For this review, take the finished solid that the model builds, in its own axes (mm). A direction names the side the tool comes from. Coordinates: 2 decimals unless noted, no trailing zeros. Loops run counter-clockwise (first coordinate to the right, second up) from the corner with the lowest first, then second, coordinate; pieces in that order, holes last. Notation, with made-up numbers: M 88,-7.75 L 123,-7.75 A20 cw 123,-1.75 Z; hole C 69,25 d3. An arc over 180 degrees is marked long. Write item = value, one per line.
from build123d import *

# Parameters (mm, degrees)
F0_R     = 2
F1_DEPTH = 32.8
F2_R     = 3
F3_DEPTH = 13.6
F4_DEPTH = 4


with BuildPart() as f1:
    # F0 (on Top) → F1 (new body)
    with BuildSketch(Plane.XY):
        with BuildLine():
            Line((77.5, 33.1), (-77.5, 33.1))
            ThreePointArc((-77.5, 33.1), (-84.571068, 30.171068), (-87.5, 23.1))
            Line((-87.5, 23.1), (-87.5, -23.1))
            ThreePointArc((-87.5, -23.1), (-84.571068, -30.171068), (-77.5, -33.1))
            Line((-77.5, -33.1), (77.5, -33.1))
            ThreePointArc((77.5, -33.1), (84.571068, -30.171068), (87.5, -23.1))
            Line((87.5, -23.1), (87.5, 23.1))
            ThreePointArc((87.5, 23.1), (84.571068, 30.171068), (77.5, 33.1))
        make_face()
        with Locations((-28.1, -20)):
            Circle(F0_R, mode=Mode.SUBTRACT)
        with Locations((71.9, -20)):
            Circle(F0_R, mode=Mode.SUBTRACT)
        with Locations((-28.1, 20)):
            Circle(F0_R, mode=Mode.SUBTRACT)
        with Locations((71.9, 20)):
            Circle(F0_R, mode=Mode.SUBTRACT)
        with Locations((-28.1, 20)):
            Circle(F0_R)
        with Locations((-28.1, -20)):
            Circle(F0_R)
        with Locations((71.9, 20)):
            Circle(F0_R)
        with Locations((71.9, -20)):
            Circle(F0_R)
    extrude(amount=F1_DEPTH)

    # F2 (on face) → F3 (join)
    with BuildSketch(Plane(origin=(-87.5, 0, 0), x_dir=(0, -1, 0), z_dir=(-1, 0, 0))):
        with Locations((0, 12)):
            Circle(F2_R)
    extrude(amount=F3_DEPTH)

    # F0 (on Top) → F4 (cut)
    with BuildSketch(Plane.XY):
        with Locations((-28.1, -20)):
            Circle(F0_R)
        with Locations((-28.1, 20)):
            Circle(F0_R)
        with Locations((71.9, 20)):
            Circle(F0_R)
        with Locations((71.9, -20)):
            Circle(F0_R)
    extrude(amount=F4_DEPTH, mode=Mode.SUBTRACT)


solid = f1.part
Q1. For pin 1 Ø1.2 at (x, y) = (-27, -20) entering from -Z; pin 2 Ø3 at (y, z) = (1.5, 25) entering from -X, all flat-tipped, find the tip position at first contact; note any pin that passes through.
Solved:
pin_1 = 4
pin_2 = -87.5
Q2. Add section B-B (y = -20). Write out the cut boundary in (x, z), and give its area (3 significant figures).
Solved:
outline = M -87.5,0 L -30.1,0 L -30.1,4 L -26.1,4 L -26.1,0 L 69.9,0 L 69.9,4 L 73.9,4 L 73.9,0 L 87.5,0 L 87.5,32.8 L -87.5,32.8 Z
area = 5,710 mm²
Q3. For line 1 along Y through (x, z) = (-28.1, 1.45); line 2 along X through (y, z) = (11, 27.5); line 3 along Y through (x, z) = (71, 1), list the stretches that pass through material, from the lowest coordinate up.
Solved:
line_1 = -33.1 to -22, -18 to 18, 22 to 33.1
line_2 = -87.5 to 87.5
line_3 = -33.1 to -21.79, -18.21 to 18.21, 21.79 to 33.1
Q4. Machinability: for faces 1 (the face through (-84.65, -30.09, 16.17)), 2 (the face through (-28, -20, 4)), 3 (the face through (-94.2, 0.65, 9.07)), which of the approach directions +Z, -Z, +X, -X, +Y, -Y give a long, thin tool a straight path to every point of the face, cutting with its end or side? Answer none if there is none.
Solved:
face_1 = +Z, -Z, -X, -Y
face_2 = -Z
face_3 = -X
Q5. Add section D-D (y = 6.5). Write out the cut boundary in (x, z), and give its area (3 significant figures).
Solved:
outline = M -87.5,0 L 87.5,0 L 87.5,32.8 L -87.5,32.8 Z
area = 5,740 mm²
Q6. Add section C-C (z = 12). Write out the cut boundary in (x, y), and give its area (3 significant figures).
Solved:
outline = M -101.1,-3 L -87.5,-3 L -87.5,-23.1 A10 ccw -77.5,-33.1 L 77.5,-33.1 A10 ccw 87.5,-23.1 L 87.5,23.1 A10 ccw 77.5,33.1 L -77.5,33.1 A10 ccw -87.5,23.1 L -87.5,3 L -101.1,3 Z
area = 11,600 mm²
Q7. Draft analysis for pull direction Y (two halves, no side actions). For faces 4 (the face through (72, -20, 4)), 5 (the face through (-101.1, 0, 12)), 6 (the face through (1, 33.1, 16)), state which applies: +Y half, -Y half, draft (parallel to the pull), parting line (faces both ways), or undercut.
Solved:
face_4 = undercut
face_5 = draft
face_6 = +Y half
Q8. Add section A-A (z = 22). Write out the cut boundary in (x, y), and give its area (3 significant figures).
Solved:
outline = M -87.5,-23.1 A10 ccw -77.5,-33.1 L 77.5,-33.1 A10 ccw 87.5,-23.1 L 87.5,23.1 A10 ccw 77.5,33.1 L -77.5,33.1 A10 ccw -87.5,23.1 Z
area = 11,500 mm²
